from build123d import *

# Parameters (mm, degrees)
SKETCH3_W            = 457.2
SKETCH3_H            = 482.6
BOSS_EXTRUDE2_DEPTH  = 5.08
SKETCH4_W            = 457.2
SKETCH4_H            = 482.6
SKETCH4_W_2          = 447.04
SKETCH4_H_2          = 472.44
BOSS_EXTRUDE3_DEPTH  = 66.04
BOSS_EXTRUDE4_DEPTH  = 66.04
BOSS_EXTRUDE5_DEPTH  = 66.04
BOSS_EXTRUDE6_DEPTH  = 66.04
BOSS_EXTRUDE7_DEPTH  = 66.04
SKETCH13_R           = 2.5
BOSS_EXTRUDE11_DEPTH = 447.04


with BuildPart() as part:
    # Sketch3 → Boss-Extrude2 (new body)
    with BuildSketch(Plane(origin=(0, 0, 0), x_dir=(1, 0, 0), z_dir=(0, 1, 0))):
        with Locations((228.6, 241.3)):
            Rectangle(SKETCH3_W, SKETCH3_H)
    extrude(amount=BOSS_EXTRUDE2_DEPTH)

    # Sketch4 → Boss-Extrude3 (add)
    with BuildSketch(Plane(origin=(0, 5.08, 0), x_dir=(1, 0, 0), z_dir=(0, 1, 0))):
        with Locations((228.6, 241.3)):
            Rectangle(SKETCH4_W, SKETCH4_H)
        with Locations((228.6, 241.3)):
            Rectangle(SKETCH4_W_2, SKETCH4_H_2, mode=Mode.SUBTRACT)
    extrude(amount=BOSS_EXTRUDE3_DEPTH)

    # Sketch5 → Boss-Extrude4 (add)
    with BuildSketch(Plane(origin=(0, 5.08, 0), x_dir=(1, 0, 0), z_dir=(0, 1, 0))):
        Polygon((5.08, 5.08), (43.208241799, 5.08), (43.208241799, 17.78), (17.78, 43.18), (5.08, 43.18), align=None)
    extrude(amount=BOSS_EXTRUDE4_DEPTH)

    # Sketch6 → Boss-Extrude5 (add)
    with BuildSketch(Plane(origin=(0, 5.08, 0), x_dir=(1, 0, 0), z_dir=(0, 1, 0))):
        Polygon((452.12, 5.08), (414.02, 5.08), (414.02, 17.78), (439.42, 43.111754401), (452.12, 43.111754401), align=None)
    extrude(amount=BOSS_EXTRUDE5_DEPTH)

    # Sketch7 → Boss-Extrude6 (add)
    with BuildSketch(Plane(origin=(0, 5.08, 0), x_dir=(1, 0, 0), z_dir=(0, 1, 0))):
        Polygon((452.12, 477.52), (452.12, 439.42), (439.42, 439.42), (414.088783751, 464.82), (414.088783751, 477.52), align=None)
    extrude(amount=BOSS_EXTRUDE6_DEPTH)

    # Sketch8 → Boss-Extrude7 (add)
    with BuildSketch(Plane(origin=(0, 5.08, 0), x_dir=(1, 0, 0), z_dir=(0, 1, 0))):
        Polygon((5.08, 477.52), (5.08, 439.42), (17.78, 439.42), (43.18, 464.82), (43.18, 477.52), align=None)
    extrude(amount=BOSS_EXTRUDE7_DEPTH)

    # Sketch13 → Boss-Extrude11 (add)
    with BuildSketch(Plane(origin=(5.08, 0, 0), x_dir=(0, 0, -1), z_dir=(1, 0, 0))):
        with Locations(Location((33.510747134, 26.94718976, 0), (0, 0, 180))):
            Circle(SKETCH13_R)
        with Locations(Location((451.021338275, 26.94718976, 0), (0, 0, 180))):
            Circle(SKETCH13_R)
    extrude(amount=BOSS_EXTRUDE11_DEPTH)


solid = part.part
The model under review builds one solid part; all positions refer to its coordinate system, in mm. A direction names the side the tool comes from. Give positions to 0.01 mm unless a question says otherwise; leave off trailing zeros. Write each loop counter-clockwise with the first axis right and the second up, starting at its lowest first coordinate (ties: lowest second). Pieces come first, ordered by that corner, then holes.
1. Tool access review of faces 1 (the flat face through (446, 38, -439.42)), 2 (the flat face through (225, 35, 0)): name each direction out of +Z, -Z, +X, -X, +Y, -Y from which nothing blocks a thin tool from reaching the whole face with its end or side.
2. Add section B-B, the plane x = 107.5. Write out the cut boundary in (y, z).
3. Wall thickness on L1, parallel to Z at x = 173.5, y = 27; L2, parallel to X at y = 26, z = -65; L3, parallel to Z at x = 269.5, y = 41: over which ranges is each line inside the solid? List them lowest first.
4. Add section A-A, the plane y = 18.5. Write out the cut boundary in (x, z).
5. For P1, Ø5, axis at x = 241, z = -323.5, coming from the +Y side, flat-tipped, find the tip position at first contact; note if it passes through.
6. Draft analysis for pull direction X (two halves, no side actions). For faces 3 (the flat face through (457.2, 35, -238)), 4 (the flat face through (225, 0, -245)), 5 (the flat face through (43.18, 38, -471)), state which applies: +X half, -X half, draft (parallel to the pull), parting line (faces both ways), or undercut.
7. Add section C-C, the plane z = -362.5. Write out the cut boundary in (x, y).
Worked answers:
1. face 1: +Y
1. face 2: +Z, +X, -X, +Y, -Y
2. outline: (0, -482.6) - (71.12, -482.6) - (71.12, -477.52) - (5.08, -477.52) - (5.08, -5.08) - (71.12, -5.08) - (71.12, 0) - (0, 0) - close; circle Ø5 at (26.95, -451.02); circle Ø5 at (26.95, -33.51)
3. L1: z = -482.6 to -477.52, -453.52 to -448.52, -36.01 to -31.01, -5.08 to 0
3. L2: x = 0 to 5.08, 452.12 to 457.2
3. L3: z = -482.6 to -477.52, -5.08 to 0
4. outline: (0, -482.6) - (457.2, -482.6) - (457.2, 0) - (0, 0) - close; hole (5.08, -439.42) - (17.78, -439.42) - (43.18, -464.82) - (43.18, -477.52) - (414.09, -477.52) - (414.09, -464.82) - (439.42, -439.42) - (452.12, -439.42) - (452.12, -43.11) - (439.42, -43.11) - (414.02, -17.78) - (414.02, -5.08) - (43.21, -5.08) - (43.21, -17.78) - (17.78, -43.18) - (5.08, -43.18) - close
5. P1: stops at y = 5.08
6. face 3: +X half
6. face 4: draft
6. face 5: undercut
7. outline: (0, 0) - (457.2, 0) - (457.2, 71.12) - (452.12, 71.12) - (452.12, 5.08) - (5.08, 5.08) - (5.08, 71.12) - (0, 71.12) - close
